Input: dimensioned drawing with shaded views. Units: mm. Origin: part minimum x, y, z. A direction names the side the tool comes from. Give positions to 0.01 mm unless a question says otherwise; leave off trailing zeros. Write each loop counter-clockwise with the first axis right and the second up, starting at its lowest first coordinate (ties: lowest second). Pieces come first, ordered by that corner, then holes.
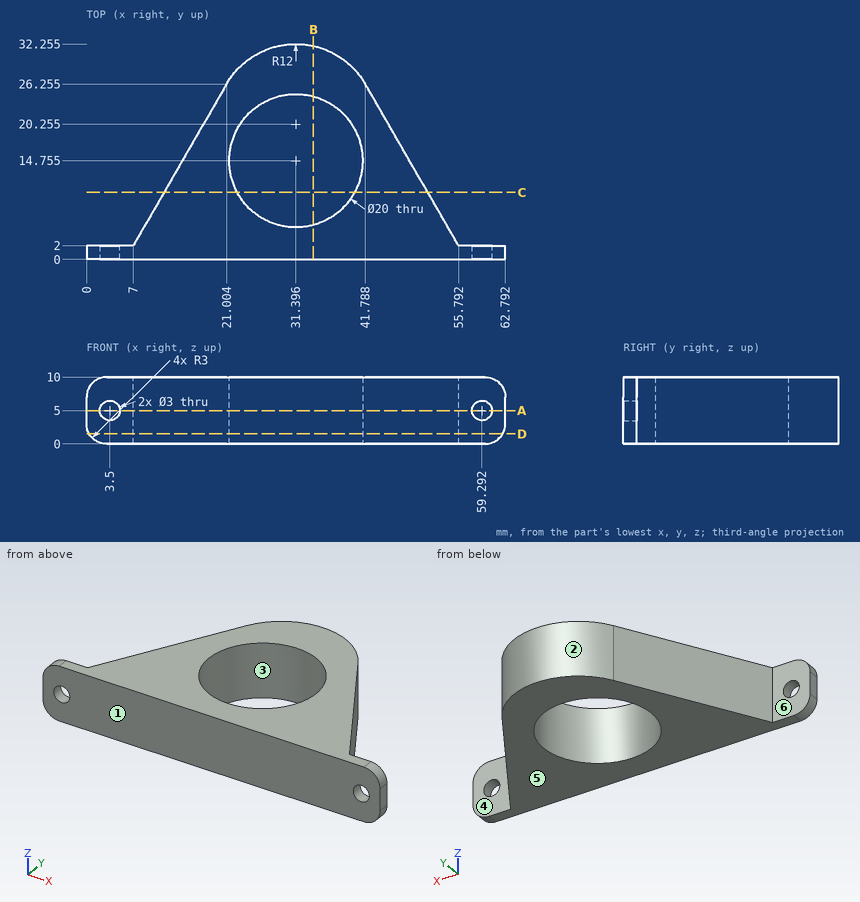
1. Mould query, pull axis X, two halves, no side actions, for the marked faces 1, 2 and 3. Classes: +X half, -X half, draft (parallel to the pull), parting line (faces both ways), or undercut.
2. Contact query for flat-ended pins moving along their axis: P1, Ø5.5, axis at x = 3, z = 4, coming from the +Y side; P2, Ø5.5, axis at x = 58, z = 7.5, coming from the +Y side; P3, Ø1, axis at x = 13.5, z = 5.5, coming from the +Y side (1 decimal); P4, Ø2.5, axis at x = 3.5, z = 5, coming from the -Y side. Output: stop coordinate, or through.
3. Cut plane A-A, the plane z = 5. Return the cut outline in (x, y) (1 decimal).
4. Line query: L1, parallel to Z at x = 3.5, y = 1.5; L2, parallel to Y at x = 25.5, z = 3.25 (1 decimal); L3, parallel to X at y = 15.5, z = 8.5 (1 decimal). Output: solid intervals per line, ascending.
5. Cut plane C-C, the plane y = 10. Return the cut outline in (x, z), then the cut area to 3 significant figures.
6. Access query for the marked faces 4, 5 and 6. Directions: +Z, -Z, +X, -X, +Y, -Y. A direction counts if a zero-diameter tool reaches every point of the face in a straight line with its end or side. Return the directions, or none.
7. Cut plane B-B, the plane x = 34. Return the cut outline in (y, z).
8. Cut plane D-D, the plane z = 1.5. Return the cut outline in (x, y) (1 decimal).
Response values:
1. face 1: draft
1. face 2: parting line
1. face 3: undercut
2. P1: stops at y = 2
2. P2: stops at y = 2.94
2. P3: stops at y = 14.1
2. P4: passes through
3. outline: (0, 0) - (2, 0) - (2, 2) - (0, 2) - close; (5, 0) - (57.8, 0) - (57.8, 2) - (55.8, 2) - (41.8, 26.3) arc R12 ccw to (21, 26.3) - (7, 2) - (5, 2) - close; (60.8, 0) - (62.8, 0) - (62.8, 2) - (60.8, 2) - close; hole circle Ø20 at (31.4, 14.8)
4. L1: z = 0 to 3.5, 6.5 to 10
4. L2: y = 0 to 6.7, 22.8 to 30.7
4. L3: x = 14.8 to 21.4, 41.4 to 48
5. outline: (11.62, 0) - (22.6, 0) - (22.6, 10) - (11.62, 10) - close; (40.19, 0) - (51.17, 0) - (51.17, 10) - (40.19, 10) - close
5. area: 220 mm2
6. face 4: +Z, -Z, +X, +Y
6. face 5: -Z, +X, -X, +Y, -Y
6. face 6: +Z, -Z, -X, +Y
7. outline: (0, 0) - (5.1, 0) - (5.1, 10) - (0, 10) - close; (24.41, 0) - (31.97, 0) - (31.97, 10) - (24.41, 10) - close
8. outline: (0.4, 0) - (62.4, 0) - (62.4, 2) - (55.8, 2) - (41.8, 26.3) arc R12 ccw to (21, 26.3) - (7, 2) - (0.4, 2) - close; hole circle Ø20 at (31.4, 14.8)
